```python
from build123d import *

# Parameters (mm, degrees)
SKETCH1_R           = 7
BOSS_EXTRUDE1_DEPTH = 10
CHAMFER1_SIZE       = 2
SKETCH2_R           = 2.4
BOSS_EXTRUDE2_DEPTH = 10


with BuildPart() as part:
    # Sketch1 → Boss-Extrude1 (new body)
    with BuildSketch(Plane(origin=(0, 0, 0), x_dir=(1, 0, 0), z_dir=(0, 1, 0))):
        with Locations(Location((0, 0, 0), (0, 0, 270))):
            Circle(SKETCH1_R)
    extrude(amount=BOSS_EXTRUDE1_DEPTH)

    # Chamfer1
    chamfer1_edges = [part.edges().sort_by_distance(p)[0] for p in [
        (0, 10, -7),
    ]]
    chamfer(chamfer1_edges, length=CHAMFER1_SIZE)

    # Sketch2 → Boss-Extrude2 (add)
    with BuildSketch(Plane(origin=(0, 10, 0), x_dir=(1, 0, 0), z_dir=(0, 1, 0))):
        with Locations(Location((0, 0, 0), (0, 0, 270))):
            Circle(SKETCH2_R)
    extrude(amount=BOSS_EXTRUDE2_DEPTH)


solid = part.part
```
For this review, take the finished solid that the model builds, in its own axes (mm). A direction names the side the tool comes from. Coordinates: 2 decimals unless noted, no trailing zeros. Order: outer loops, then holes, each group sorted by start corner. A loop starts at its lowest first (then second) coordinate and runs counter-clockwise, first axis right, second up. Notation, with made-up numbers: (-10, 44.5) - (22, 44.5) arc R31 cw to (22, 73.5) - close; hole circle Ø4 at (16.5, 63). An arc over 180 degrees is marked (long way). Answer as a JSON object with one key per item and string values. Group by question number.
1. We need section D-D on y = 11. State the section outline as (x, z) points, then the cut area to 3 significant figures.
2. For probe 1 along Y at (x, z) = (1.25, 3.75); probe 2 along Z at (x, y) = (5.5, 3.5); probe 3 along X at (y, z) = (8.75, -3.25), list the stretches that pass through material, from the lowest coordinate up.
3. We need section B-B on z = 0. State the section outline as (x, y) points, then the cut area to 3 significant figures.
4. Clearance check with flat-ended pins moving along their axes: P1, Ø1.5, axis at x = -3.5, y = 5, coming from the +Z side; P2, Ø1, axis at y = 7, z = -4.5, coming from the +X side; P3, Ø5, axis at y = 17, z = 0, coming from the +X side. State where each tip first meets the part, or that it passes through.
5. We need section C-C on y = 4. State the section outline as (x, z) points.
6. We need section A-A on x = 0. State the section outline as (y, z) points.
7. For faces 1 (the flat face through (2.3, 10, -1.2)), 2 (the flat face through (0, 0, 0)), list the 3-axis set-ups (+Z, -Z, +X, -X, +Y, -Y) from which the entire face can be reached by the end or side of a thin tool; tool diameter is ignored.
Final values:
{
 "1": {"outline": "circle Ø4.8 at (0, 0)", "area": "18.1 mm²"},
 "2": {"probe 1": "0 to 10", "probe 2": "-4.33 to 4.33", "probe 3": "-5.34 to 5.34"},
 "3": {"outline": "(-7, 0) - (7, 0) - (7, 8) - (5, 10) - (2.4, 10) - (2.4, 20) - (-2.4, 20) - (-2.4, 10) - (-5, 10) - (-7, 8) - close", "area": "184 mm²"},
 "4": {"P1": "z = 6.44", "P2": "x = 5.74", "P3": "x = 2.4"},
 "5": {"outline": "circle Ø14 at (0, 0)"},
 "6": {"outline": "(0, -7) - (8, -7) - (10, -5) - (10, -2.4) - (20, -2.4) - (20, 2.4) - (10, 2.4) - (10, 5) - (8, 7) - (0, 7) - close"},
 "7": {"face 1": "+Y", "face 2": "+Z, -Z, +X, -X, -Y"}
}
